Geometry check sheet. Reference: the model listing, model coordinates, mm. A direction names the side the tool comes from. Round coordinates to 2 decimals unless told otherwise and drop trailing zeros. Write each loop counter-clockwise with the first axis right and the second up, starting at its lowest first coordinate (ties: lowest second). Pieces come first, ordered by that corner, then holes. Notation, with made-up numbers: (45, -13) -> (63, -13) arc R12 cw to (63, 0) -> close; hole circle Ø11 at (78.25, 16.5). An arc over 180 degrees is marked (long way). One line per question, with ' | ' between items.
Autodesk Inventor part; units mm, degrees
ref_plane "YZ Plane" through (0, 0, 0) normal (1, 0, 0) x (0, 1, 0)
ref_plane "XZ Plane" through (0, 0, 0) normal (0, 1, 0) x (-1, 0, 0)
ref_plane "XY Plane" through (0, 0, 0) normal (0, 0, 1) x (1, 0, 0)
sketch "Sketch3" plane through (0, 0, 0) normal (0, 0, 1) x (1, 0, 0)
  circle A0 centre (0, 0) radius 4.7625
  circle A1 centre (0, 0) radius 3.175
  dimension "d4" = 9.525
  dimension "d5" = 6.35
extrude "Extrusion2" add sketch "Sketch3" along normal blind 143.51 contours A0 | A1
extrude "Extrusion3" cut sketch "Sketch3" along normal blind 13.2055
sketch "Sketch4" plane through (0, 0, 143.51) normal (0, 0, 1) x (1, 0, 0)
  circle A0 centre (0, 0) radius 3.175
  line L0 (0, -7.1984) -> (-6.234, -3.5992)
  line L1 (-6.234, -3.5992) -> (-6.234, 3.5992)
  line L2 (-6.234, 3.5992) -> (0, 7.1984)
  line L3 (0, 7.1984) -> (6.234, 3.5992)
  line L4 (6.234, 3.5992) -> (6.234, -3.5992)
  line L5 (6.234, -3.5992) -> (0, -7.1984)
  dimension "d10" = 14.3967
extrude "Extrusion4" add sketch "Sketch4" against normal blind 122.6287
properties part number "hex rod"
(1) Sectioned sample at A-A on y = 0. Record the cut outline in (x, z) (1 decimal), then the cut area to 3 significant figures.
Resolved:
outline: (-6.2, 20.9) -> (-4.8, 20.9) -> (-4.8, 13.2) -> (-3.2, 13.2) -> (-3.2, 0) -> (3.2, 0) -> (3.2, 13.2) -> (4.8, 13.2) -> (4.8, 20.9) -> (6.2, 20.9) -> (6.2, 143.5) -> (-6.2, 143.5) -> close | area: 1,690 mm2
(2) Go/stop test with flat-tipped pins: pin 1 (6 mm diameter, centred on x = -2.5, y = 1.5, fed in from -Z); pin 2 (1.5 mm diameter, centred on x = 5, z = 38.5, fed in from -Y). Record where each tip stops, or that it passes through.
Resolved:
pin 1: stops at z = 0 | pin 2: stops at y = -4.74
(3) Sectioned sample at B-B on z = 27.5. Record the cut outline in (x, y), then the cut area to 3 significant figures.
Resolved:
outline: (-6.23, -3.6) -> (0, -7.2) -> (6.23, -3.6) -> (6.23, 3.6) -> (0, 7.2) -> (-6.23, 3.6) -> close | area: 135 mm2
(4) Access from +Z, -Z, +X, -X, +Y, -Y to the whole of each face (thin tool, end or side, straight path). Record for faces 1 (the flat face through (3.161, -5.374, 83.054)), 2 (the cylindrical face through (-3.78, 2.9, 16.99)).
Resolved:
face 1: +Z, -Z, +X, -Y | face 2: -Z
(5) Material ranges on line 1 (Z direction, x = -2.25, y = -2.5); line 2 (Y direction, x = 4.25, z = 119); line 3 (Z direction, x = -4, y = -4.75), recorded low to high.
Resolved:
line 1: z = 13.21 to 143.51 | line 2: y = -4.74 to 4.74 | line 3: z = 20.88 to 143.51
